Part model, mm, in its own coordinate system. Coordinates: 2 decimals unless noted, no trailing zeros. Loops run counter-clockwise (first coordinate to the right, second up) from the corner with the lowest first, then second, coordinate; pieces in that order, holes last. Notation, with made-up numbers: (19.25, 17) -> (26.25, 17) arc R15 cw to (26.25, 27) -> close; hole circle Ø3 at (86.5, -27). An arc over 180 degrees is marked (long way). One line per question, with ' | ' between items. Start each with the question number.
1) Drop flat-ended pins along their axis: pin 1 (6 mm diameter, centred on x = -0.5, y = 1.5, fed in from +Z); pin 2 (4 mm diameter, centred on x = -4.5, z = 31, fed in from +Y). Give the stop position or say it passes through.
2) Cut at C-C (y = 4.25). List the corners of the cut face in (x, z), plus the area to 3 significant figures.
3) Cut at D-D (x = 4.5). List the corners of the cut face in (y, z), plus the area to 3 significant figures.
4) Cut at A-A (x = -1.25). List the corners of the cut face in (y, z).
5) Probe L1, parallel to Y at x = -0.25, z = 31; L2, parallel to X at y = 0.25, z = 42.5; L3, parallel to X at y = 2, z = 3.5. List the from-to ranges inside material, lowest first. Write a range as from..to.
from build123d import *

# Parameters (mm, degrees)
F0_R     = 1.5
F1_DEPTH = 50


# Not quite as in the source:
# - ends of sketch curves that miss each other by under 0.0002 mm in the source are joined


with BuildPart() as f1:
    # F0 (on Top) → F1 (new body)
    with BuildSketch(Plane.XY):
        with BuildLine():
            Line((-5.449118, -0.504862), (-4.441162, -5.402211))
            ThreePointArc((-4.441162, -5.402211), (0.6615584195, -4.0525834634), (5.5830371113, -2.1451512457))
            Line((5.5830371113, -2.1451512457), (3.519902, 2.409349))
            Line((3.519902, 2.409349), (3.498846, 2.399818))
            ThreePointArc((3.498846, 2.399818), (0.6786519051, 5.1349674747), (-3.2332818366, 4.772594717))
            ThreePointArc((-3.2332818366, 4.772594717), (-5.2226446667, 2.5075404986), (-5.4264814855, -0.5001971285))
            Line((-5.4264814855, -0.5001971285), (-5.449118, -0.504862))
        make_face()
        with Locations((-0.883526, 0.702699)):
            Circle(F0_R, mode=Mode.SUBTRACT)
    extrude(amount=F1_DEPTH)


solid = f1.part
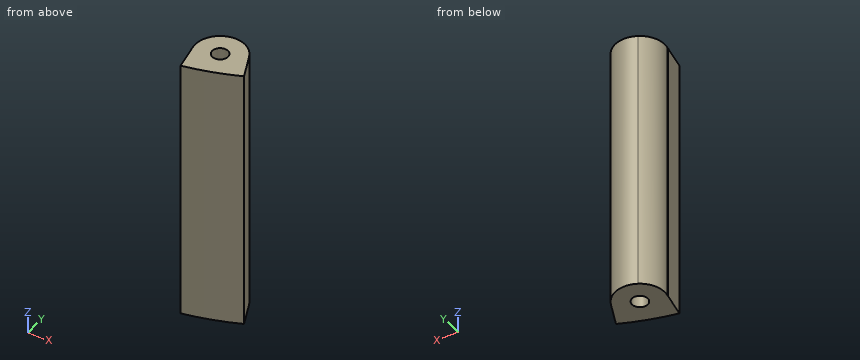
Reported:
1) pin 1: stops at z = 50 | pin 2: stops at y = 5.12
2) outline: (-3.97, 0) -> (2.2, 0) -> (2.2, 50) -> (-3.97, 50) -> close | area: 308 mm²
3) outline: (-2.62, 0) -> (0.25, 0) -> (0.25, 50) -> (-2.62, 50) -> close | area: 143 mm²
4) outline: (-4.63, 0) -> (-0.75, 0) -> (-0.75, 50) -> (-4.63, 50) -> close; (2.16, 0) -> (5.39, 0) -> (5.39, 50) -> (2.16, 50) -> close
5) L1: y = -4.34..-0.66, 2.06..5.36 | L2: x = -5.56..-2.31, 0.55..4.5 | L3: x = -5.4..-1.64, -0.13..3.71
